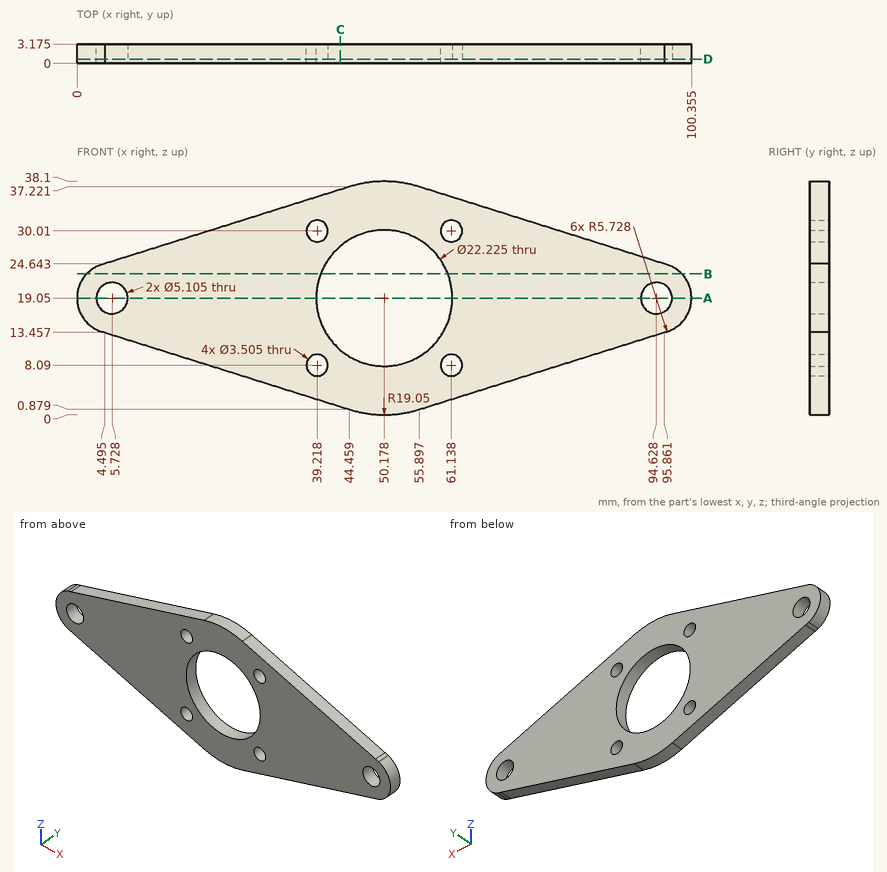
The figure shows three views and two pictorial views of one solid part (mm, origin at its lowest corner). Answer the questions. Round coordinates to 2 decimals unless told otherwise and drop trailing zeros. Write each loop counter-clockwise with the first axis right and the second up, starting at its lowest first coordinate (ties: lowest second). Pieces come first, ordered by that corner, then holes. Notation, with made-up numbers: M 69.5,70.5 L 102.5,70.5 A13 ccw 102.5,90.5 Z; hole C -31,55.25 d11. An arc over 180 degrees is marked long. Write each question's results on one line, items separated by ' | '. Start each with the question number.
(1) Find the intervals of material crossed by line 1 (X direction, y = 2.75, z = 19.5) (1 decimal); line 2 (Z direction, x = 40.5, y = 1.2) (1 decimal); line 3 (Z direction, x = 4, y = 0.65), in increasing order.
(2) The part is cut by section D-D, the plane y = 0.7. Give the number of separate pieces and of enclosed holes in the cut face, and give its area (3 significant figures).
(3) The part is cut by section C-C, the plane x = 43. Write down the section's boundary in (y, z) (1 decimal).
(4) The part is cut by section A-A, the plane z = 19.05. Write down the section's boundary in (x, y) (1 decimal).
(5) The part is cut by section B-B, the plane z = 23. Write down the section's boundary in (x, y) (1 decimal).
(6) Each of these flat-tipped pins is pushed along its axis until it touches: P1, Ø2, axis at x = 39.22, z = 30.01, coming from the +Y side; P2, Ø4, axis at x = 41, z = 13, coming from the -Y side; P3, Ø1, axis at y = 0.5, z = 15.5, coming from the -X side. Where does it stop, or does it pass through?
Worked answers:
1) line 1: x = 0 to 3.2, 8.2 to 39.1, 61.3 to 92.1, 97.1 to 100.3 | line 2: z = 2.1 to 6.9, 9.3 to 13.6, 24.5 to 28.8, 31.2 to 36 | line 3: z = 13.59 to 17.17, 20.93 to 24.51
2) separate pieces: 1 | enclosed holes: 7 | area: 1,940 mm²
3) outline: M 0,1.3 L 3.2,1.3 L 3.2,10.6 L 0,10.6 Z; M 0,27.5 L 3.2,27.5 L 3.2,36.8 L 0,36.8 Z
4) outline: M 0,0 L 3.2,0 L 3.2,3.2 L 0,3.2 Z; M 8.3,0 L 39.1,0 L 39.1,3.2 L 8.3,3.2 Z; M 61.3,0 L 92.1,0 L 92.1,3.2 L 61.3,3.2 Z; M 97.2,0 L 100.4,0 L 100.4,3.2 L 97.2,3.2 Z
5) outline: M 1.6,0 L 39.8,0 L 39.8,3.2 L 1.6,3.2 Z; M 60.6,0 L 98.8,0 L 98.8,3.2 L 60.6,3.2 Z
6) P1: passes through | P2: stops at y = 0 | P3: stops at x = 0.88
